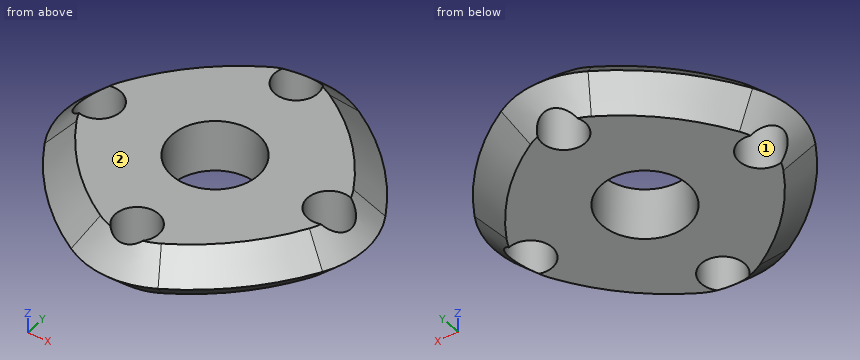
from build123d import *

# Parameters (mm, degrees)
F0_W         = 50.8
F0_H         = 50.8
F0_R         = 6.35
F1_DEPTH     = 7.62
F2_T1_DEPTH  = 198.12
F4_D         = 6.35
F5_R         = 12.7
F6_T2_ANGLE  = 29.9999999999
F6_T4_ANGLE  = 29.9999999999
F6_T6_ANGLE  = 60.000000035
F6_T8_ANGLE  = 60.000000035
F6_T10_ANGLE = 29.9999999999
F6_T12_ANGLE = 60.000000035
F6_T14_ANGLE = 29.9999999999
F6_T16_ANGLE = 60.000000035
F6_T18_ANGLE = 29.9999999999
F6_T20_ANGLE = 60.000000035
F6_T22_ANGLE = 60.000000035
F6_T24_ANGLE = 29.9999999999
F6_T26_ANGLE = 60.000000035
F6_T28_ANGLE = 29.9999999999
F6_T30_ANGLE = 60.000000035
F6_T32_ANGLE = 29.9999999999


# Not quite as in the source:
# - a fillet or chamfer that OpenCascade refuses, or shapes differently, is made with other operations: its cross-section is extruded or revolved along the edge and cut away or added


with BuildPart() as f1:
    # F0 (on Top) → F1 (new body)
    with BuildSketch(Plane.XY):
        Rectangle(F0_W, F0_H)
        Circle(F0_R, mode=Mode.SUBTRACT)
    extrude(amount=F1_DEPTH)

    # F2: fillet of radius 38.1 on 4 edges, made by hand

    # F2_s2 → F2_t1 (cut)
    with BuildSketch(Plane.XY.offset(-95.25)):
        with BuildLine():
            ThreePointArc((25.4, 12.7), (14.2407683632, -14.2407683632), (-12.7, -25.4))
            Line((-12.7, -25.4), (25.4, -25.4))
            Line((25.4, -25.4), (25.4, 12.7))
        make_face()
        with BuildLine():
            ThreePointArc((-25.4, 12.7), (-14.2407683632, -14.2407683632), (12.7, -25.4))
            Line((12.7, -25.4), (-25.4, -25.4))
            Line((-25.4, -25.4), (-25.4, 12.7))
        make_face()
        with BuildLine():
            ThreePointArc((12.7, 25.4), (-14.2407683632, 14.2407683632), (-25.4, -12.7))
            Line((-25.4, -12.7), (-25.4, 25.4))
            Line((-25.4, 25.4), (12.7, 25.4))
        make_face()
        with BuildLine():
            ThreePointArc((25.4, -12.7), (14.2407683632, 14.2407683632), (-12.7, 25.4))
            Line((-12.7, 25.4), (25.4, 25.4))
            Line((25.4, 25.4), (25.4, -12.7))
        make_face()
    extrude(amount=F2_T1_DEPTH, mode=Mode.SUBTRACT)

    # F4 (through all)
    with Locations(Plane(origin=(0, 0, 0), x_dir=(1, 0, 0), z_dir=(0, 0, -1))):
        with Locations((0, -16.4350587875), (-16.9112086296, 0), (0, 15.7412625849), (16.6794583201, 0)):
            Hole(F4_D / 2)

    # F5
    f5_edges = [f1.edges().sort_by_distance(p)[0] for p in [
        (0, -23.221024, 3.81),
        (23.221024, 0, 3.81),
        (-23.221024, 0, 3.81),
        (0, 23.221024, 3.81),
    ]]
    fillet(f5_edges, radius=F5_R)

    # F6: chamfer of 3.81 on 2 edges, made by hand

    # F6_s1 → F6_t2 (revolve, cut)
    with BuildSketch(Plane(origin=(2.324261314, 4.025738686, 0), x_dir=(0, 0, 1), z_dir=(0.5, 0.8660254038, 0))):
        Polygon((3.81, 20.7514773719), (7.62, 16.9414773719), (7.62, 20.7514773719), align=None)
    revolve(axis=Axis((-12.7, 12.7, 7.62), (0, 0, -1)), revolution_arc=F6_T2_ANGLE, mode=Mode.SUBTRACT)

    # F6_s3 → F6_t4 (revolve, cut)
    with BuildSketch(Plane(origin=(2.324261314, 4.025738686, 0), x_dir=(0, 0, 1), z_dir=(0.5, 0.8660254038, 0))):
        Polygon((0, 16.9414773719), (3.81, 20.7514773719), (0, 20.7514773719), align=None)
    revolve(axis=Axis((-12.7, 12.7, 0), (0, 0, -1)), revolution_arc=F6_T4_ANGLE, mode=Mode.SUBTRACT)

    # F6_s5 → F6_t6 (revolve, cut)
    with BuildSketch(Plane(origin=(2.324261317, -4.0257386892, 0), x_dir=(0, 0, 1), z_dir=(-0.5000000002, 0.8660254037, 0))):
        Polygon((0, 16.941477371), (3.81, 20.7514773707), (0, 20.751477371), align=None)
    revolve(axis=Axis((9.2970452639, 1.5e-09, 0), (0, 0, -1)), revolution_arc=F6_T6_ANGLE, mode=Mode.SUBTRACT)

    # F6_s7 → F6_t8 (revolve, cut)
    with BuildSketch(Plane(origin=(4.0257386892, -2.324261317, 0), x_dir=(0, 0, 1), z_dir=(-0.8660254037, 0.5000000002, 0))):
        Polygon((0, -16.941477371), (3.81, -20.7514773707), (0, -20.751477371), align=None)
    revolve(axis=Axis((-1.5e-09, -9.2970452639, 0), (0, 0, 1)), revolution_arc=F6_T8_ANGLE, mode=Mode.SUBTRACT)

    # F6_s9 → F6_t10 (revolve, cut)
    with BuildSketch(Plane(origin=(4.025738686, -2.324261314, 0), x_dir=(0, 0, 1), z_dir=(0.8660254038, -0.5, 0))):
        Polygon((0, 16.9414773719), (3.81, 20.7514773719), (0, 20.7514773719), align=None)
    revolve(axis=Axis((12.7, 12.7, 0), (0, 0, -1)), revolution_arc=F6_T10_ANGLE, mode=Mode.SUBTRACT)

    # F6_s11 → F6_t12 (revolve, cut)
    with BuildSketch(Plane(origin=(-2.324261317, -4.0257386892, 0), x_dir=(0, 0, 1), z_dir=(0.5000000002, 0.8660254037, 0))):
        Polygon((0, -16.941477371), (3.81, -20.7514773707), (0, -20.751477371), align=None)
    revolve(axis=Axis((-9.2970452639, 1.5e-09, 0), (0, 0, 1)), revolution_arc=F6_T12_ANGLE, mode=Mode.SUBTRACT)

    # F6_s13 → F6_t14 (revolve, cut)
    with BuildSketch(Plane(origin=(-2.324261314, -4.025738686, 0), x_dir=(0, 0, 1), z_dir=(-0.5, -0.8660254038, 0))):
        Polygon((0, 16.9414773719), (3.81, 20.7514773719), (0, 20.7514773719), align=None)
    revolve(axis=Axis((12.7, -12.7, 0), (0, 0, -1)), revolution_arc=F6_T14_ANGLE, mode=Mode.SUBTRACT)

    # F6_s15 → F6_t16 (revolve, cut)
    with BuildSketch(Plane(origin=(4.0257386892, 2.324261317, 0), x_dir=(0, 0, 1), z_dir=(-0.8660254037, -0.5000000002, 0))):
        Polygon((0, 16.941477371), (3.81, 20.7514773707), (0, 20.751477371), align=None)
    revolve(axis=Axis((-1.5e-09, 9.2970452639, 0), (0, 0, -1)), revolution_arc=F6_T16_ANGLE, mode=Mode.SUBTRACT)

    # F6_s17 → F6_t18 (revolve, cut)
    with BuildSketch(Plane(origin=(-4.025738686, 2.324261314, 0), x_dir=(0, 0, 1), z_dir=(-0.8660254038, 0.5, 0))):
        Polygon((0, 16.9414773719), (3.81, 20.7514773719), (0, 20.7514773719), align=None)
    revolve(axis=Axis((-12.7, -12.7, 0), (0, 0, -1)), revolution_arc=F6_T18_ANGLE, mode=Mode.SUBTRACT)

    # F6_s19 → F6_t20 (revolve, cut)
    with BuildSketch(Plane(origin=(2.324261317, -4.0257386892, 0), x_dir=(0, 0, 1), z_dir=(-0.5000000002, 0.8660254037, 0))):
        Polygon((3.81, 20.7514773707), (7.62, 16.941477371), (7.62, 20.751477371), align=None)
    revolve(axis=Axis((9.2970452639, 1.5e-09, 7.62), (0, 0, -1)), revolution_arc=F6_T20_ANGLE, mode=Mode.SUBTRACT)

    # F6_s21 → F6_t22 (revolve, cut)
    with BuildSketch(Plane(origin=(4.0257386892, -2.324261317, 0), x_dir=(0, 0, 1), z_dir=(-0.8660254037, 0.5000000002, 0))):
        Polygon((3.81, -20.7514773707), (7.62, -16.941477371), (7.62, -20.751477371), align=None)
    revolve(axis=Axis((-1.5e-09, -9.2970452639, 7.62), (0, 0, 1)), revolution_arc=F6_T22_ANGLE, mode=Mode.SUBTRACT)

    # F6_s23 → F6_t24 (revolve, cut)
    with BuildSketch(Plane(origin=(4.025738686, -2.324261314, 0), x_dir=(0, 0, 1), z_dir=(0.8660254038, -0.5, 0))):
        Polygon((3.81, 20.7514773719), (7.62, 16.9414773719), (7.62, 20.7514773719), align=None)
    revolve(axis=Axis((12.7, 12.7, 7.62), (0, 0, -1)), revolution_arc=F6_T24_ANGLE, mode=Mode.SUBTRACT)

    # F6_s25 → F6_t26 (revolve, cut)
    with BuildSketch(Plane(origin=(-2.324261317, -4.0257386892, 0), x_dir=(0, 0, 1), z_dir=(0.5000000002, 0.8660254037, 0))):
        Polygon((3.81, -20.7514773707), (7.62, -16.941477371), (7.62, -20.751477371), align=None)
    revolve(axis=Axis((-9.2970452639, 1.5e-09, 7.62), (0, 0, 1)), revolution_arc=F6_T26_ANGLE, mode=Mode.SUBTRACT)

    # F6_s27 → F6_t28 (revolve, cut)
    with BuildSketch(Plane(origin=(-2.324261314, -4.025738686, 0), x_dir=(0, 0, 1), z_dir=(-0.5, -0.8660254038, 0))):
        Polygon((3.81, 20.7514773719), (7.62, 16.9414773719), (7.62, 20.7514773719), align=None)
    revolve(axis=Axis((12.7, -12.7, 7.62), (0, 0, -1)), revolution_arc=F6_T28_ANGLE, mode=Mode.SUBTRACT)

    # F6_s29 → F6_t30 (revolve, cut)
    with BuildSketch(Plane(origin=(4.0257386892, 2.324261317, 0), x_dir=(0, 0, 1), z_dir=(-0.8660254037, -0.5000000002, 0))):
        Polygon((3.81, 20.7514773707), (7.62, 16.941477371), (7.62, 20.751477371), align=None)
    revolve(axis=Axis((-1.5e-09, 9.2970452639, 7.62), (0, 0, -1)), revolution_arc=F6_T30_ANGLE, mode=Mode.SUBTRACT)

    # F6_s31 → F6_t32 (revolve, cut)
    with BuildSketch(Plane(origin=(-4.025738686, 2.324261314, 0), x_dir=(0, 0, 1), z_dir=(-0.8660254038, 0.5, 0))):
        Polygon((3.81, 20.7514773719), (7.62, 16.9414773719), (7.62, 20.7514773719), align=None)
    revolve(axis=Axis((-12.7, -12.7, 7.62), (0, 0, -1)), revolution_arc=F6_T32_ANGLE, mode=Mode.SUBTRACT)


solid = f1.part
Design review of the part built by this model. Coordinates are the model's own, in mm. Face numbers are marked on the shaded views. Round coordinates to 2 decimals unless told otherwise and drop trailing zeros. Write each loop counter-clockwise with the first axis right and the second up, starting at its lowest first coordinate (ties: lowest second). Pieces come first, ordered by that corner, then holes. Notation, with made-up numbers: (80, -28) - (102, -28) arc R28 ccw to (102, 7) - close; hole circle Ø11 at (73.25, 33.5). An arc over 180 degrees is marked (long way). Use a Markdown table: item, result. Add a question column.
1. Clearance check with flat-ended pins moving along their axes: pin 1 (8.5 mm diameter, centred on x = 0, y = 16.44, fed in from +Z); pin 2 (2 mm diameter, centred on y = 1.5, z = 4.5, fed in from -X); pin 3 (10 mm diameter, centred on x = 0, y = 0, fed in from +Z); pin 4 (2 mm diameter, centred on x = 0, z = 2, fed in from +Y). State where each tip first meets the part, or that it passes through.
2. Wall thickness on probe 1 along Y at (x, z) = (0, 4.5); probe 2 along Y at (x, z) = (0, 3); probe 3 along Y at (x, z) = (1.5, 1): over which ranges is each line inside the solid? List them lowest first.
3. Mouldability with a two-part tool opening along X and no side actions: class the marked faces 1 and 2 as +X half, -X half, draft (parallel to the pull), parting line (faces both ways), or undercut.
4. We need section B-B (x = 0). State the section outline as (y, z) points, then the cut area to 3 significant figures.
5. We need section A-A (y = 0). State the section outline as (x, z) points.
Output:
| question | item | result |
|---|---|---|
| 1 | pin 1 | stops at z = 7.62 |
| 1 | pin 2 | stops at x = -21.97 |
| 1 | pin 3 | passes through |
| 1 | pin 4 | stops at y = 21.19 |
| 2 | probe 1 | y = -21.31 to -18.92, -12.57 to -6.35, 6.35 to 13.26, 19.61 to 21.31 |
| 2 | probe 2 | y = -21.19 to -18.92, -12.57 to -6.35, 6.35 to 13.26, 19.61 to 21.19 |
| 2 | probe 3 | y = -19.07 to -18.54, -12.94 to -6.17, 6.17 to 13.64 |
| 3 | face 1 | undercut |
| 3 | face 2 | draft |
| 4 | outline | (-22, 3.81) - (-18.92, 0.73) - (-18.92, 6.89) - close; (-12.57, 0) - (-6.35, 0) - (-6.35, 7.62) - (-12.57, 7.62) - close; (6.35, 0) - (13.26, 0) - (13.26, 7.62) - (6.35, 7.62) - close; (19.61, 1.42) - (22, 3.81) - (19.61, 6.2) - close |
| 4 | area | 115 mm2 |
| 5 | outline | (-22, 3.81) - (-20.09, 1.9) - (-20.09, 5.72) - close; (-13.74, 0) - (-6.35, 0) - (-6.35, 7.62) - (-13.74, 7.62) - close; (6.35, 0) - (13.5, 0) - (13.5, 7.62) - (6.35, 7.62) - close; (19.85, 1.67) - (22, 3.81) - (19.85, 5.95) - close |
